Input: part model. Units: mm. Frame: model coordinates. A direction names the side the tool comes from. Give positions to 0.01 mm unless a question says otherwise; leave off trailing zeros. Loops run counter-clockwise (first coordinate to the right, second up) from the corner with the lowest first, then second, coordinate; pieces in that order, holes last. Notation, with made-up numbers: M -17,-36.5 L 29,-36.5 A9 ccw 29,-30.5 Z; hole C 79.25,-37 d10. An arc over 180 degrees is marked long. One line per item, written item: value. Start each with the question number.
(1) Pull-direction query (Z, two-part tool) for faces 5 (the flat face through (3, 2.297, 31)), 6 (the flat face through (3, 7, 7)); classes: released by +Z, released by -Z, zero draft, split by the parting line, or undercut.
(2) Section A-A on z = 17.5. Output: boundary loops of the cut face in (x, y).
(3) Section B-B on y = 3.25. State how many separate pieces and enclosed holes the cut face has, plus the area to 3 significant figures.
(4) Pin query (flat end, axial travel): P1, Ø5, axis at y = 4.5, z = 14, coming from the +X side; P2, Ø4, axis at x = 1.5, z = 5, coming from the -Y side; P3, Ø1, axis at y = -5, z = 1, coming from the -X side. Return the tip coordinate at first contact, or that it passes through.
(5) Access query for faces 1 (the flat face through (17, -5.703, 16)), 2 (the flat face through (-9, 0, 17)), 3 (the flat face through (3, 7, 25)), 4 (the flat face through (-8.208, -1, 31)). Directions: +Z, -Z, +X, -X, +Y, -Y. A direction counts if a zero-diameter tool reaches every point of the face in a straight line with its end or side. Return the directions, or none.
(6) Ray query, line 1 along Y through (x, z) = (-7, 30.5); line 2 along Z through (x, y) = (1, -6.5); line 3 along X through (y, z) = (7.25, 23). Return the intervals inside material, ascending. Write a range as from..to.
(7) Section C-C on z = 11.5. Output: boundary loops of the cut face in (x, y).
```python
from build123d import *

# Parameters (mm, degrees)
BOSS_EXTRUDE1_DEPTH = 32
SKETCH2_W           = 22
SKETCH2_H           = 2
BOSS_EXTRUDE2_DEPTH = 14
SKETCH4_W           = 3
SKETCH4_H           = 11
CUT_EXTRUDE2_DEPTH  = 45.506992773
LPATTERN1_COUNT     = 6
LPATTERN1_PITCH     = 5
SKETCH5_W           = 22
SKETCH5_H           = 3
CUT_EXTRUDE3_DEPTH  = 40.853893963
LPATTERN2_COUNT     = 6
LPATTERN2_PITCH     = 5
SKETCH6_W           = 22
SKETCH6_H           = 2
CUT_EXTRUDE4_DEPTH  = 37.567270471
LPATTERN3_COUNT     = 3
LPATTERN3_PITCH     = 4
BOSS_EXTRUDE3_DEPTH = 2.4


with BuildPart() as part:
    # Sketch1 → Boss-Extrude1 (new body)
    with BuildSketch(Plane.XY):
        Polygon((-13.608, -5.703470261), (-13.608, -8.103470261), (-8.208, -8.103470261), (-8.208, 5.896529739), (13.792, 5.896529739), (13.792, -8.103470261), (19.192, -8.103470261), (19.192, -5.703470261), (16.192, -5.703470261), (16.192, 8.296529739), (-10.608, 8.296529739), (-10.608, -5.703470261), align=None)
    extrude(amount=BOSS_EXTRUDE1_DEPTH)

    # Sketch2 → Boss-Extrude2 (add)
    with BuildSketch(Plane.XZ.offset(-5.896529739)):
        with Locations((2.792, 31)):
            Rectangle(SKETCH2_W, SKETCH2_H)
        with Locations((2.792, 1)):
            Rectangle(SKETCH2_W, SKETCH2_H)
    extrude(amount=BOSS_EXTRUDE2_DEPTH)

    # Sketch4 → Cut-Extrude2 (cut, through all)
    with BuildSketch(Plane.ZY.offset(10.608)):
        with Locations((28.5, -0.203470261)):
            Rectangle(SKETCH4_W, SKETCH4_H)
    cut_extrude2 = extrude(amount=-CUT_EXTRUDE2_DEPTH, mode=Mode.SUBTRACT)

    # LPattern1: Cut-Extrude2 ×6
    with Locations(*[(0, 0, -i * LPATTERN1_PITCH) for i in range(1, LPATTERN1_COUNT)]):
        add(cut_extrude2, mode=Mode.SUBTRACT)

    # Sketch5 → Cut-Extrude3 (cut, through all)
    with BuildSketch(Plane.XZ.offset(-5.896529739)):
        with Locations((2.792, 28.5)):
            Rectangle(SKETCH5_W, SKETCH5_H)
    cut_extrude3 = extrude(amount=-CUT_EXTRUDE3_DEPTH, mode=Mode.SUBTRACT)

    # LPattern2: Cut-Extrude3 ×6
    with Locations(*[(0, 0, -i * LPATTERN2_PITCH) for i in range(1, LPATTERN2_COUNT)]):
        add(cut_extrude3, mode=Mode.SUBTRACT)

    # Sketch6 → Cut-Extrude4 (cut, symmetric)
    with BuildSketch(Plane(origin=(0, 0, 30), x_dir=(-1, 0, 0), z_dir=(0, 0, -1))):
        with Locations((-2.792, -4.703470261)):
            Rectangle(SKETCH6_W, SKETCH6_H)
    cut_extrude4 = extrude(amount=CUT_EXTRUDE4_DEPTH, both=True, mode=Mode.SUBTRACT)

    # LPattern3: Cut-Extrude4 ×3
    with Locations(*[(0, i * LPATTERN3_PITCH, 0) for i in range(1, LPATTERN3_COUNT)]):
        add(cut_extrude4, mode=Mode.SUBTRACT)

    # Sketch8 → Boss-Extrude3 (add)
    with BuildSketch(Plane.XZ.offset(8.103470261)):
        Polygon((-13.608, 30), (-14.008, 30.4), (-14.008, 31.6), (-13.608, 32), align=None)
        Polygon((-13.608, 2), (-13.608, 0), (-14.008, 0.4), (-14.008, 1.6), align=None)
        Polygon((19.192, 2), (19.592, 1.6), (19.592, 0.4), (19.192, 0), align=None)
        Polygon((19.192, 30), (19.192, 32), (19.592, 31.6), (19.592, 30.4), align=None)
    extrude(amount=-BOSS_EXTRUDE3_DEPTH)


solid = part.part
```
Output values:
1. face 5: zero draft
1. face 6: undercut
2. outline: M -13.61,-8.1 L -8.21,-8.1 L -8.21,-5.7 L -13.61,-5.7 Z; M -10.61,5.3 L -8.21,5.3 L -8.21,8.3 L -10.61,8.3 Z; M 13.79,-8.1 L 19.19,-8.1 L 19.19,-5.7 L 13.79,-5.7 Z; M 13.79,5.3 L 16.19,5.3 L 16.19,8.3 L 13.79,8.3 Z
3. separate pieces: 14
3. enclosed holes: 0
3. area: 67.2 mm²
4. P1: stops at x = 16.19
4. P2: stops at y = 5.9
4. P3: stops at x = -10.61
5. face 1: +X
5. face 2: +X, -X
5. face 3: +Y, -Y
5. face 4: +Z, -Z
6. line 1: y = -8.1..-5.7, -3.7..-1.7, 0.3..2.3, 4.3..8.3
6. line 2: z = 0..2, 30..32
6. line 3: x = -10.61..-8.21, 13.79..16.19
7. outline: M -13.61,-8.1 L -8.21,-8.1 L -8.21,5.9 L 13.79,5.9 L 13.79,-8.1 L 19.19,-8.1 L 19.19,-5.7 L 16.19,-5.7 L 16.19,8.3 L -10.61,8.3 L -10.61,-5.7 L -13.61,-5.7 Z
